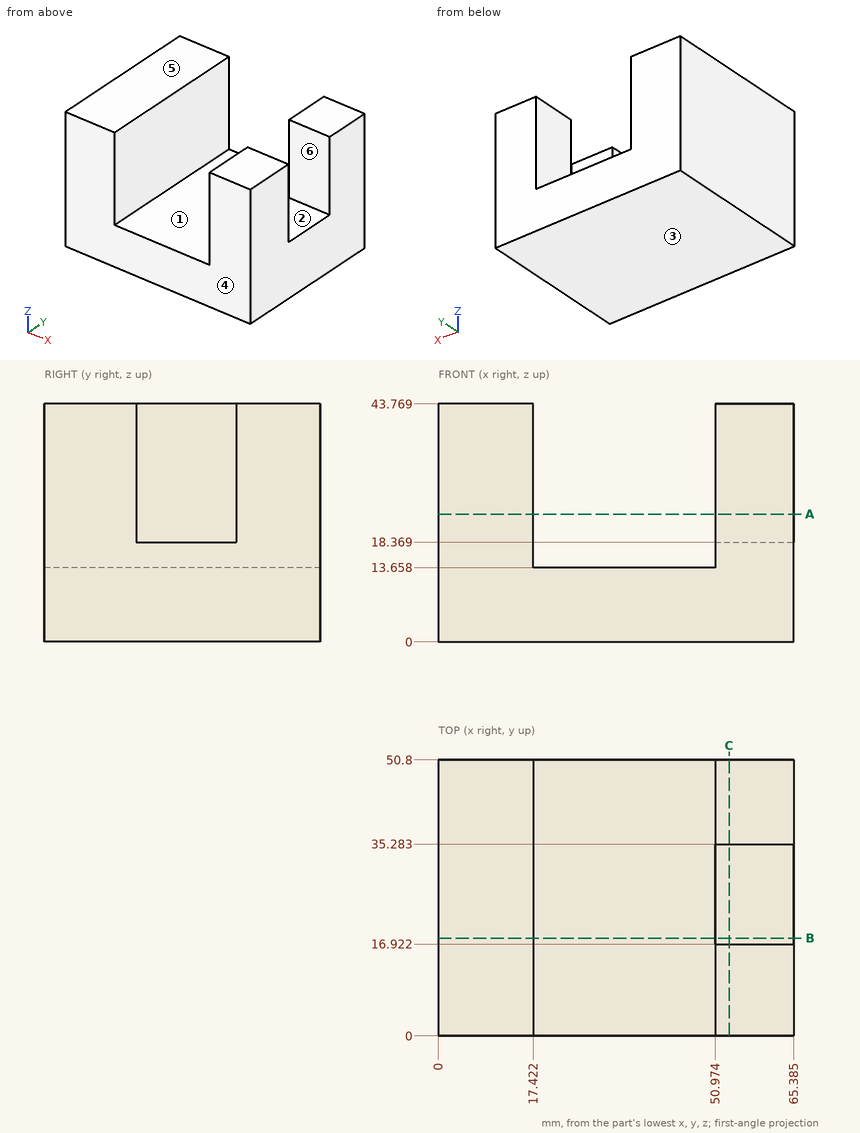
Input: dimensioned drawing with shaded views. Units: mm. Origin: part minimum x, y, z. A direction names the side the tool comes from. Round coordinates to 2 decimals unless told otherwise and drop trailing zeros. Loops run counter-clockwise (first coordinate to the right, second up) from the corner with the lowest first, then second, coordinate; pieces in that order, holes last. Notation, with made-up numbers: (72.5, -18) -> (84.5, -18) arc R15 cw to (84.5, -14) -> close; hole circle Ø10 at (-19.75, 79). An arc over 180 degrees is marked (long way). Answer as a JSON object with one key per item and string values. Group by question number.
Q1. Section query B-B (y = 18). Output: boundary loops of the cut face in (x, z) (1 decimal).
Q2. Section query A-A (z = 23.5). Output: boundary loops of the cut face in (x, y) (1 decimal).
Q3. Mould query, pull axis Y, two halves, no side actions, for the marked faces 4, 5 and 6. Classes: pulls with the +Y half, pulls with the -Y half, needs draft (parallel to the pull), parting line crosses it, or undercut.
Q4. Section query C-C (x = 53.5). Output: boundary loops of the cut face in (y, z).
Q5. Access query for the marked faces 1, 2 and 3. Directions: +Z, -Z, +X, -X, +Y, -Y. A direction counts if a zero-diameter tool reaches every point of the face in a straight line with its end or side. Return the directions, or none.
Q6. Ray query, line 1 (X direction, y = 2, z = 34.5) (1 decimal); line 2 (Y direction, x = 56, z = 19.5); line 3 (Z direction, x = 38, y = 18.5). Return the intervals inside material, ascending. Write a range as from..to.
Q7. Contact query for flat-ended pins moving along their axis: P1, Ø5, axis at x = 23.5, y = 30.5, coming from the +Z side; P2, Ø7, axis at x = 56.5, y = 29.5, coming from the +Z side. Output: stop coordinate, or through.
Completed:
{
 "1": {"outline": "(0, 0) -> (65.4, 0) -> (65.4, 18.4) -> (51, 18.4) -> (51, 13.7) -> (17.4, 13.7) -> (17.4, 43.8) -> (0, 43.8) -> close"},
 "2": {"outline": "(0, 0) -> (17.4, 0) -> (17.4, 50.8) -> (0, 50.8) -> close; (51, 0) -> (65.4, 0) -> (65.4, 16.9) -> (51, 16.9) -> close; (51, 35.3) -> (65.4, 35.3) -> (65.4, 50.8) -> (51, 50.8) -> close"},
 "3": {"face 4": "pulls with the -Y half", "face 5": "needs draft", "face 6": "undercut"},
 "4": {"outline": "(0, 0) -> (50.8, 0) -> (50.8, 43.77) -> (35.28, 43.77) -> (35.28, 18.37) -> (16.92, 18.37) -> (16.92, 43.77) -> (0, 43.77) -> close"},
 "5": {"face 1": "+Z, +Y, -Y", "face 2": "+Z, +X", "face 3": "-Z, +X, -X, +Y, -Y"},
 "6": {"line 1": "0..17.4, 51..65.4", "line 2": "0..16.92, 35.28..50.8", "line 3": "0..13.66"},
 "7": {"P1": "z = 13.66", "P2": "z = 18.37"}
}
